Source: CAD feature listing. Evaluate the final solid. Frame: model axes, mm. Round coordinates to 2 decimals unless told otherwise and drop trailing zeros. Order: outer loops, then holes, each group sorted by start corner. A loop starts at its lowest first (then second) coordinate and runs counter-clockwise, first axis right, second up. Notation, with made-up numbers: M 43,-21 L 96,-21 A15 cw 96,-5 Z; hole C 68.5,61.5 d5. An arc over 180 degrees is marked long. Use one line per item in the form item = value. Start each with the question number.
Q1. Section C-C (y = 209). Return the cut outline in (x, z).
Q2. Contact query for flat-ended pins moving along their axis: pin 1 (1 mm diameter, centred on x = 1, z = -41, fed in from -Y); pin 2 (11.5 mm diameter, centred on y = -27.78, z = -23.81, fed in from -X). Output: stop coordinate, or through.
Q3. Section B-B (z = -36). Return the cut outline in (x, y).
Q4. Material intervals for probe 1 along Z at (x, y) = (-0.5, -31); probe 2 along Z at (x, y) = (-0.5, 33.5); probe 3 along Z at (x, y) = (-0.25, 95.5), sorted ascending.
Q5. Pull-direction query (Y, two-part tool) for faces 1 (the cylindrical face through (-0.022, -21.915, -26.245)), 2 (the flat face through (0.02, 150.63, 26.8)), 3 (the flat face through (1.588, 57, -3)); classes: pulls with the +Y half, pulls with the -Y half, needs draft (parallel to the pull), parting line crosses it, or undercut.
from build123d import *

# Parameters (mm, degrees)
F0_R     = 6.35
F1_DEPTH = 1.5875
F2_R     = 1.5875


with BuildPart() as f1:
    # F0 (on Right) → F1 (new body, symmetric)
    with BuildSketch(Plane.YZ):
        with BuildLine():
            ThreePointArc((51.196875, -23.8125), (32.7506622905, 25.8960511115), (-13.6571946485, 51.5380797221))
            ThreePointArc((-13.6571946485, 51.5380797221), (-74.7116761115, 33.9412872905), (-101.203125, -23.8125))
            ThreePointArc((-101.203125, -23.8125), (-98.8413616364, -42.6368143416), (-91.9024738075, -60.2942369259))
            Line((-91.9024738075, -60.2942369259), (0, -48.815625))
            Line((0, -48.815625), (0, -23.415625))
            Line((0, -23.415625), (3.175, -23.415625))
            Line((3.175, -23.415625), (3.175, -48.3443618613))
            Line((3.175, -48.3443618613), (49.1093522758, -41.5263564983))
            ThreePointArc((49.1093522758, -41.5263564983), (50.6731948379, -32.730718196), (51.196875, -23.8125))
        make_face()
        with Locations((-27.78125, -23.8125)):
            Circle(F0_R, mode=Mode.SUBTRACT)
        with BuildLine():
            ThreePointArc((310.3672615954, -2.7480187483), (307.1812515299, 0.0029156046), (310.3730287107, 2.7471565524))
            Line((310.3730287107, 2.7471565524), (-13.6571946485, 51.5380797221))
            ThreePointArc((-13.6571946485, 51.5380797221), (32.7506622905, 25.8960511115), (51.196875, -23.8125))
            ThreePointArc((51.196875, -23.8125), (50.6731948379, -32.730718196), (49.1093522758, -41.5263564983))
            Line((49.1093522758, -41.5263564983), (310.3672615954, -2.7480187483))
        make_face()
        with BuildLine():
            ThreePointArc((310.3672615954, -2.7480187483), (312.0630786939, -1.8144997338), (312.7375, 0))
            ThreePointArc((312.7375, 0), (312.0649818283, 1.8122909259), (310.3730287107, 2.7471565524))
            ThreePointArc((310.3730287107, 2.7471565524), (307.1812515299, 0.0029156046), (310.3672615954, -2.7480187483))
        make_face()
        Polygon((0, -48.815625), (3.175, -48.3443618613), (3.175, -23.415625), (0, -23.415625), align=None)
    extrude(amount=F1_DEPTH, both=True)

    # F2
    f2_edges = [f1.edges().sort_by_distance(p)[0] for p in [
        (0, -91.902474, -60.294237),
    ]]
    fillet(f2_edges, radius=F2_R)


solid = f1.part
Results list:
q1.outline = M -1.59,-17.79 L 1.59,-17.79 L 1.59,18.01 L -1.59,18.01 Z
q2.pin_1 = -99.35
q2.pin_2 = through
q3.outline = M -1.59,-100.22 L 1.59,-100.22 L 1.59,86.34 L -1.59,86.34 Z
q4.probe_1 = -52.69 to -29.29, -18.34 to 52.15
q4.probe_2 = -43.84 to 44.44
q4.probe_3 = -34.64 to 35.1
q5.face_1 = undercut
q5.face_2 = pulls with the +Y half
q5.face_3 = needs draft
